The listing builds one solid part. Answer for the finished solid, in the listing's coordinates (mm). A direction names the side the tool comes from. Give positions to 0.01 mm unless a question says otherwise; leave off trailing zeros. Write each loop counter-clockwise with the first axis right and the second up, starting at its lowest first coordinate (ties: lowest second). Pieces come first, ordered by that corner, then holes. Notation, with made-up numbers: M -25,81.25 L 26,81.25 A12 cw 26,85.25 Z; hole C 26,53.5 d8. An arc over 180 degrees is marked long. Answer as a JSON object with one key per item and string values.
Autodesk Inventor part; units mm, degrees
ref_plane "YZ Plane" through (0, 0, 0) normal (1, 0, 0) x (0, 1, 0)
ref_plane "XZ Plane" through (0, 0, 0) normal (0, 1, 0) x (-1, 0, 0)
ref_plane "XY Plane" through (0, 0, 0) normal (0, 0, 1) x (1, 0, 0)
sketch "Sketch1" plane through (0, 0, 0) normal (1, 0, 0) x (0, 1, 0)
  line L0 (0, 0) -> (0, -12)
  line L1 (0, -12) -> (20, -12)
  line L2 (20, -12) -> (20, -18)
  line L3 (20, -18) -> (0, -18)
  line L4 (0, -18) -> (0, -30)
  line L5 (1.5, 0) -> (1.5, -10.5)
  line L6 (1.5, -10.5) -> (21.5, -10.5)
  line L7 (21.5, -10.5) -> (21.5, -19.5)
  line L8 (21.5, -19.5) -> (1.5, -19.5)
  line L9 (1.5, -19.5) -> (1.5, -30)
  line L10 (1.5, 0) -> (0, 0)
  line L11 (1.5, -30) -> (0, -30)
  dimension "d0" = 12
  dimension "d1" = 12
  dimension "d2" = 6
  dimension "d3" = 20
  dimension "d4" = 1.5
extrude "Extrusion1" add sketch "Sketch1" along normal blind 8
sketch "Sketch2" plane through (0, 1.5, 0) normal (0, 1, 0) x (1, 0, 0)
  line L0 (0, 0) -> (8, 0) construction
  line L1 (0, 10.5) -> (0, 0) construction
  line L2 (0, 30) -> (0, 19.5) construction
  point P0 (4, 5.25)
  point P1 (4, 24.75)
  point P2 (0, 5.25)
  point P3 (0, 24.75)
  point P4 (4, 0)
  point P5 (4, 0)
hole "Hole1" at (4, 1.5, -5.25) at (4, 1.5, -24.75) direction (0, -1, 0) diameter 4 end through all countersink diameter 5 countersink angle 90
fillet "Fillet1" radius 0.5 12 edges at (4, 21.5, -10.5) (4, 21.5, -19.5) (4, 20, -12) (4, 20, -18) (4, 0, -12) (4, 0, -18) (4, 1.5, -10.5) (4, 1.5, -19.5) (4, 1.5, -30) (4, 0, -30) (4, 1.5, 0) (4, 0, 0)
properties part number "CLIP V1"
1. A cutting plane is placed at C-C, the plane x = 4. Count the separate pieces of the cut face and the enclosed holes in it, plus the area to 3 significant figures.
Verdict:
{"separate pieces": "3", "enclosed holes": "0", "area": "92.3 mm2"}
2. A cutting plane is placed at B-B, the plane z = -5.25. Give the vertices of the cut face in (x, y).
Verdict:
{"outline": "M 0,0 L 2,0 L 2,1 L 1.5,1.5 L 0,1.5 Z; M 6,0 L 8,0 L 8,1.5 L 6.5,1.5 L 6,1 Z"}
3. Flat-ended cylindrical pins translate along their axes: pin 1 (3 mm diameter, centred on x = 5.5, y = 10.5, fed in from -Z); pin 2 (4 mm diameter, centred on x = 5, z = -24, fed in from +Y); pin 3 (2.5 mm diameter, centred on x = 5.5, z = -14, fed in from -Y). Find the tip coordinate at first contact, or state that the pin passes through.
Verdict:
{"pin 1": "stops at z = -19.5", "pin 2": "stops at y = 1.5", "pin 3": "stops at y = 20"}
4. A cutting plane is placed at D-D, the plane x = 7.5. Give the vertices of the cut face in (y, z), plus the area to 3 significant figures.
Verdict:
{"outline": "M 0,-29.5 A0.5 ccw 0.5,-30 L 1,-30 A0.5 ccw 1.5,-29.5 L 1.5,-20 A0.5 cw 2,-19.5 L 21,-19.5 A0.5 ccw 21.5,-19 L 21.5,-11 A0.5 ccw 21,-10.5 L 2,-10.5 A0.5 cw 1.5,-10 L 1.5,-0.5 A0.5 ccw 1,0 L 0.5,0 A0.5 ccw 0,-0.5 L 0,-11.5 A0.5 ccw 0.5,-12 L 19.5,-12 A0.5 cw 20,-12.5 L 20,-17.5 A0.5 cw 19.5,-18 L 0.5,-18 A0.5 ccw 0,-18.5 Z", "area": "105 mm2"}
5. Consider line 1 along Z through (x, y) = (4, 0.5); line 2 along Z through (x, y) = (4.75, 18.25); line 3 along X through (y, z) = (0.8, -24.75). Determine where each line is inside the solid, lowest interval first.
Verdict:
{"line 1": "z = -30 to -26.75, -22.75 to -18, -12 to -7.25, -3.25 to 0", "line 2": "z = -19.5 to -18, -12 to -10.5", "line 3": "x = 0 to 2, 6 to 8"}
6. The mould has two halves that part along Z. Classify faces 5 (the flat face through (4, 10, -12)), 6 (the flat face through (4, 11, -10.5)), 7 (the flat face through (0, 8.3, -18.3)), 8 (the cylindrical face through (5.217, 0.493, -6.837)): released by +Z, released by -Z, zero draft, split by the parting line, or undercut.
Verdict:
{"face 5": "undercut", "face 6": "released by +Z", "face 7": "zero draft", "face 8": "undercut"}
7. For faces 1 (the flat face through (4, 20, -15)), 2 (the flat face through (4, 12, -19.5)), 3 (the flat face through (3.1, 0, -22.7)), 4 (the flat face through (7, 1.5, -5)), determine the directions among +Z, -Z, +X, -X, +Y, -Y from which every point of the face is accessible in a straight line to the end or side of a thin tool.
Verdict:
{"face 1": "+X, -X, -Y", "face 2": "-Z, +X, -X, +Y", "face 3": "+Z, -Z, +X, -X, -Y", "face 4": "+Z, +X, -X, +Y"}
8. A cutting plane is placed at A-A, the plane y = 7.5. Give the vertices of the cut face in (x, z).
Verdict:
{"outline": "M 0,-19.5 L 8,-19.5 L 8,-18 L 0,-18 Z; M 0,-12 L 8,-12 L 8,-10.5 L 0,-10.5 Z"}
